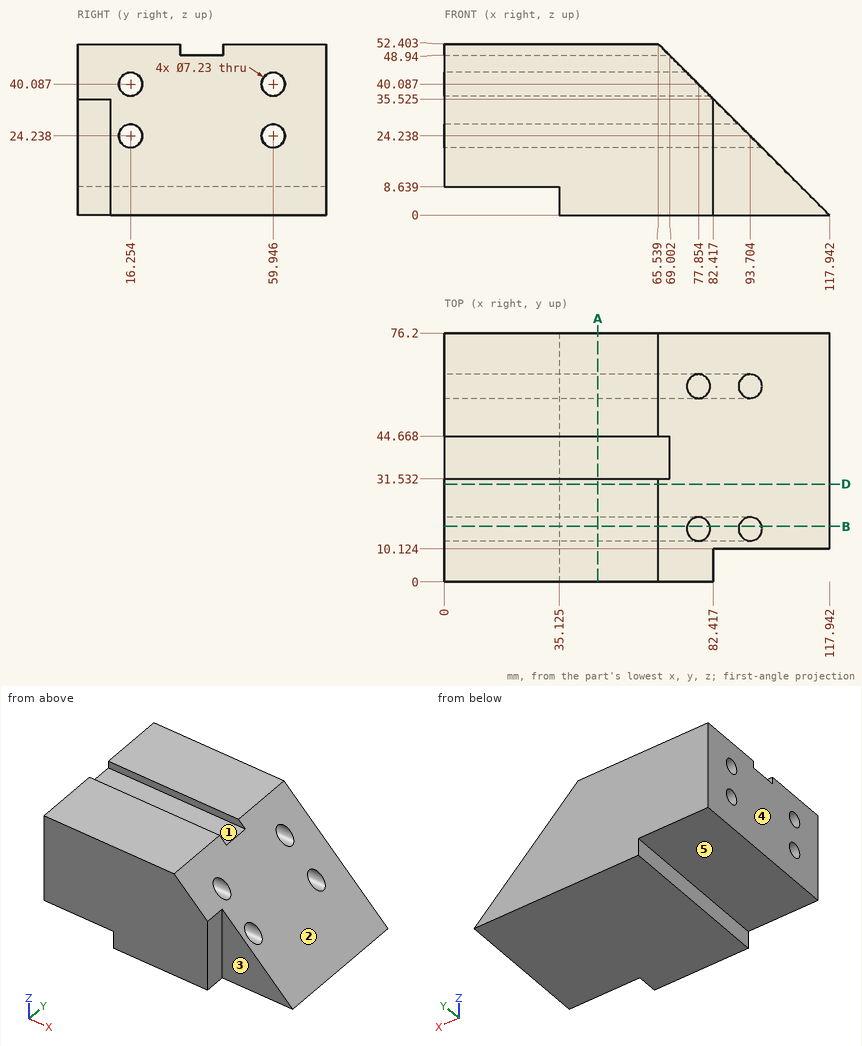
Could you check a few things on this drawing? It's one solid part, dimensions in mm from its lowest x, y, z. A direction names the side the tool comes from. Coordinates: 2 decimals unless noted, no trailing zeros. Order: outer loops, then holes, each group sorted by start corner. A loop starts at its lowest first (then second) coordinate and runs counter-clockwise, first axis right, second up. Notation, with made-up numbers: M 62.25,72.25 L 90.25,72.25 A37 ccw 90.25,111.25 Z; hole C 42,5 d9. An arc over 180 degrees is marked long. Use a Markdown table: item, result. Add a question column.
Q1. If I drill on L1, parallel to Y at x = 9, z = 43 (1 decimal); L2, parallel to Y at x = 37, z = 42 (1 decimal); L3, parallel to Z at x = 54.5, y = 42.5, over which ranges is the centre line in solid material (lowest first)?
Q2. Which directions (+Z, -Z, +X, -X, +Y, -Y) give clear straight access to the entire face, cutting with the end or side of a thin tool? Please do the marked faces 4 and 5.
Q3. I'm going to push flat-ended pins straight in: pin 1 (10.5 mm diameter, centred on x = 107, z = 15, fed in from -Y); pin 2 (4 mm diameter, centred on x = 51, y = 41.5, fed in from +Z); pin 3 (10.5 mm diameter, centred on x = 20, y = 40.5, fed in from -Z). Where does each tip first touch, or does it pass through?
Q4. I want a section at B-B on y = 17. Give the number of separate pieces and of enclosed holes in the cut face, then the cut area to 3 significant figures.
Q5. I want a section at A-A on x = 47. List the corners of the cut face in (y, z) for me (1 decimal).
Q6. I want a section at D-D on y = 30. List the corners of the cut face in (x, z) for me (1 decimal).
Q7. We'd pull the mould along Y, two halves only. Please class the marked faces 1, 2 and 3: pulls with the +Y half, pulls with the -Y half, needs draft (parallel to the pull), parting line crosses it, or undercut.
Checked values:
| question | item | result |
|---|---|---|
| 1 | L1 | 0 to 14.1, 18.4 to 57.8, 62.1 to 76.2 |
| 1 | L2 | 0 to 13.2, 19.3 to 56.9, 63 to 76.2 |
| 1 | L3 | 0 to 48.94 |
| 2 | face 4 | +Z, -Z, -X, +Y, -Y |
| 2 | face 5 | -Z, -X, +Y, -Y |
| 3 | pin 1 | y = 10.12 |
| 3 | pin 2 | z = 48.94 |
| 3 | pin 3 | z = 8.64 |
| 4 | separate pieces | 3 |
| 4 | enclosed holes | 0 |
| 4 | area | 3,290 mm² |
| 5 | outline | M 0,0 L 76.2,0 L 76.2,52.4 L 44.7,52.4 L 44.7,48.9 L 31.5,48.9 L 31.5,52.4 L 0,52.4 Z; hole C 16.3,24.2 d7.2; hole C 16.3,40.1 d7.2; hole C 59.9,24.2 d7.2; hole C 59.9,40.1 d7.2 |
| 6 | outline | M 0,8.6 L 35.1,8.6 L 35.1,0 L 117.9,0 L 65.5,52.4 L 0,52.4 Z |
| 7 | face 1 | undercut |
| 7 | face 2 | needs draft |
| 7 | face 3 | pulls with the -Y half |
